```python
from build123d import *

# Parameters (mm, degrees)
SKETCH1_W           = 159.1
SKETCH1_H           = 45
BOSS_EXTRUDE1_DEPTH = 5.9
BOSS_EXTRUDE3_DEPTH = 5.9
CUT_EXTRUDE1_REACH  = 7.9
SKETCH4_R           = 2.05


with BuildPart() as part:
    # Sketch1 → Boss-Extrude1 (new body)
    with BuildSketch(Plane.XY):
        Rectangle(SKETCH1_W, SKETCH1_H)
    extrude(amount=BOSS_EXTRUDE1_DEPTH)

    # Sketch3 → Boss-Extrude3 (add)
    with BuildSketch(Plane.XY.offset(5.9)):
        Polygon((-79.55, 7.5), (-85.45, 7.5), (-85.45, 12.5), (-93.45, 12.5), (-93.45, -2.5), (-85.45, -2.5), (-79.55, -2.5), align=None)
        Polygon((79.55, -2.5), (79.55, 7.5), (85.45, 7.5), (85.45, 12.5), (93.45, 12.5), (93.45, -2.5), (85.45, -2.5), align=None)
    extrude(amount=-BOSS_EXTRUDE3_DEPTH)

    # Sketch4 → Cut-Extrude1 (cut, up to next)
    with BuildSketch(Plane.XY.offset(5.9), mode=Mode.PRIVATE) as cut_extrude1_sk1:
        with Locations((-79.55, 7.5)):
            Circle(SKETCH4_R)
    cut_extrude1_tool1 = extrude(cut_extrude1_sk1.sketch, amount=-CUT_EXTRUDE1_REACH, mode=Mode.PRIVATE) & part.part
    add(cut_extrude1_tool1.solids().sort_by_distance((-79.55, 7.5, 5.9))[0], mode=Mode.SUBTRACT)
    # Sketch4 → Cut-Extrude1 (cut, up to next)
    with BuildSketch(Plane.XY.offset(5.9), mode=Mode.PRIVATE) as cut_extrude1_sk2:
        with Locations((-79.55, -2.5)):
            Circle(SKETCH4_R)
    cut_extrude1_tool2 = extrude(cut_extrude1_sk2.sketch, amount=-CUT_EXTRUDE1_REACH, mode=Mode.PRIVATE) & part.part
    add(cut_extrude1_tool2.solids().sort_by_distance((-79.55, -2.5, 5.9))[0], mode=Mode.SUBTRACT)
    # Sketch4 → Cut-Extrude1 (cut, up to next)
    with BuildSketch(Plane.XY.offset(5.9), mode=Mode.PRIVATE) as cut_extrude1_sk3:
        with Locations((79.55, -2.5)):
            Circle(SKETCH4_R)
    cut_extrude1_tool3 = extrude(cut_extrude1_sk3.sketch, amount=-CUT_EXTRUDE1_REACH, mode=Mode.PRIVATE) & part.part
    add(cut_extrude1_tool3.solids().sort_by_distance((79.55, -2.5, 5.9))[0], mode=Mode.SUBTRACT)
    # Sketch4 → Cut-Extrude1 (cut, up to next)
    with BuildSketch(Plane.XY.offset(5.9), mode=Mode.PRIVATE) as cut_extrude1_sk4:
        with Locations((79.55, 7.5)):
            Circle(SKETCH4_R)
    cut_extrude1_tool4 = extrude(cut_extrude1_sk4.sketch, amount=-CUT_EXTRUDE1_REACH, mode=Mode.PRIVATE) & part.part
    add(cut_extrude1_tool4.solids().sort_by_distance((79.55, 7.5, 5.9))[0], mode=Mode.SUBTRACT)
    # Sketch4 → Cut-Extrude1 (cut, up to next)
    with BuildSketch(Plane.XY.offset(5.9), mode=Mode.PRIVATE) as cut_extrude1_sk5:
        with Locations((-85.45, 7.5)):
            Circle(SKETCH4_R)
    cut_extrude1_tool5 = extrude(cut_extrude1_sk5.sketch, amount=-CUT_EXTRUDE1_REACH, mode=Mode.PRIVATE) & part.part
    add(cut_extrude1_tool5.solids().sort_by_distance((-85.45, 7.5, 5.9))[0], mode=Mode.SUBTRACT)
    # Sketch4 → Cut-Extrude1 (cut, up to next)
    with BuildSketch(Plane.XY.offset(5.9), mode=Mode.PRIVATE) as cut_extrude1_sk6:
        with Locations((85.45, 7.5)):
            Circle(SKETCH4_R)
    cut_extrude1_tool6 = extrude(cut_extrude1_sk6.sketch, amount=-CUT_EXTRUDE1_REACH, mode=Mode.PRIVATE) & part.part
    add(cut_extrude1_tool6.solids().sort_by_distance((85.45, 7.5, 5.9))[0], mode=Mode.SUBTRACT)


solid = part.part
```
Model file for the job. Use its own axes, mm. A direction names the side the tool comes from. Round coordinates to 2 decimals unless told otherwise and drop trailing zeros. Order: outer loops, then holes, each group sorted by start corner. A loop starts at its lowest first (then second) coordinate and runs counter-clockwise, first axis right, second up. Notation, with made-up numbers: (-15.5, 7) -> (40.5, 7) arc R9 ccw to (40.5, 23) -> close; hole circle Ø1 at (2, 37). An arc over 180 degrees is marked (long way). Use one line per item in the form item = value.
Item 1: Pull direction Y, two halves, no side cores. Call faces 1 (the face through (-1, 0, 5.9)), 2 (the face through (87, -2.5, 3)), 3 (the face through (86.85, 6, 2.99)): released by +Y, released by -Y, zero draft, split by the parting line, or undercut.
Returned:
face_1 = zero draft
face_2 = released by -Y
face_3 = undercut
Item 2: Tool access for faces 4 (the face through (89, 12.5, 3)), 5 (the face through (-89, 12.5, 3)), 6 (the face through (79.55, -14, 3)), 7 (the face through (-88, -2.5, 3)), 8 (the face through (79.55, 16, 3)): list every direction of +Z, -Z, +X, -X, +Y, -Y with a clear straight run to the whole face (end or side of a thin tool).
Returned:
face_4 = +Z, -Z, +X, +Y
face_5 = +Z, -Z, -X, +Y
face_6 = +Z, -Z, +X, -Y
face_7 = +Z, -Z, -X, -Y
face_8 = +Z, -Z, +Y
Item 3: Cut at A-A, the plane z = 1.05. Write the cut outline in (x, y), and give its area (3 significant figures).
Returned:
outline = (-93.45, -2.5) -> (-81.6, -2.5) arc R2.05 cw (long way) to (-79.55, -4.55) -> (-79.55, -22.5) -> (79.55, -22.5) -> (79.55, -4.55) arc R2.05 cw (long way) to (81.6, -2.5) -> (93.45, -2.5) -> (93.45, 12.5) -> (85.45, 12.5) -> (85.45, 9.55) arc R2.05 cw (long way) to (83.4, 7.5) -> (81.6, 7.5) arc R2.05 cw (long way) to (79.55, 9.55) -> (79.55, 22.5) -> (-79.55, 22.5) -> (-79.55, 9.55) arc R2.05 cw (long way) to (-81.6, 7.5) -> (-83.4, 7.5) arc R2.05 cw (long way) to (-85.45, 9.55) -> (-85.45, 12.5) -> (-93.45, 12.5) -> close
area = 7,460 mm^2
Item 4: Drill centre lines: line 1 (X direction, y = 8, z = 2.6); line 2 (X direction, y = -6.5, z = 3.55); line 3 (X direction, y = 7, z = 3). Where is each one in solid material? Low to high.
Returned:
line_1 = -93.45 to -87.44, -77.56 to 77.56, 87.44 to 93.45
line_2 = -79.55 to 79.55
line_3 = -93.45 to -87.44, -83.46 to -81.54, -77.56 to 77.56, 81.54 to 83.46, 87.44 to 93.45
Item 5: Flat gauge pins, fed straight in: pin 1 Ø2 at (x, z) = (83, 3) entering from +Y; pin 2 Ø1.8 at (y, z) = (17, 3) entering from +X; pin 3 Ø3 at (y, z) = (-14.5, 3.5) entering from +X; pin 4 Ø3.5 at (x, y) = (-79.55, 7.5) entering from +Z. Where does each tip first touch, or does it go through?
Returned:
pin_1 = 7.5
pin_2 = 79.55
pin_3 = 79.55
pin_4 = through
Item 6: Cut at B-B, the plane y = -10.5. Write the cut outline in (x, z).
Returned:
outline = (-79.55, 0) -> (79.55, 0) -> (79.55, 5.9) -> (-79.55, 5.9) -> close
